Answer from the drawing. Dimensions are ordinates in mm from the lowest x, y and z of the part. A direction names the side the tool comes from. Give positions to 0.01 mm unless a question says otherwise; leave off trailing zeros. Order: outer loops, then holes, each group sorted by start corner. A loop starts at its lowest first (then second) coordinate and runs counter-clockwise, first axis right, second up.
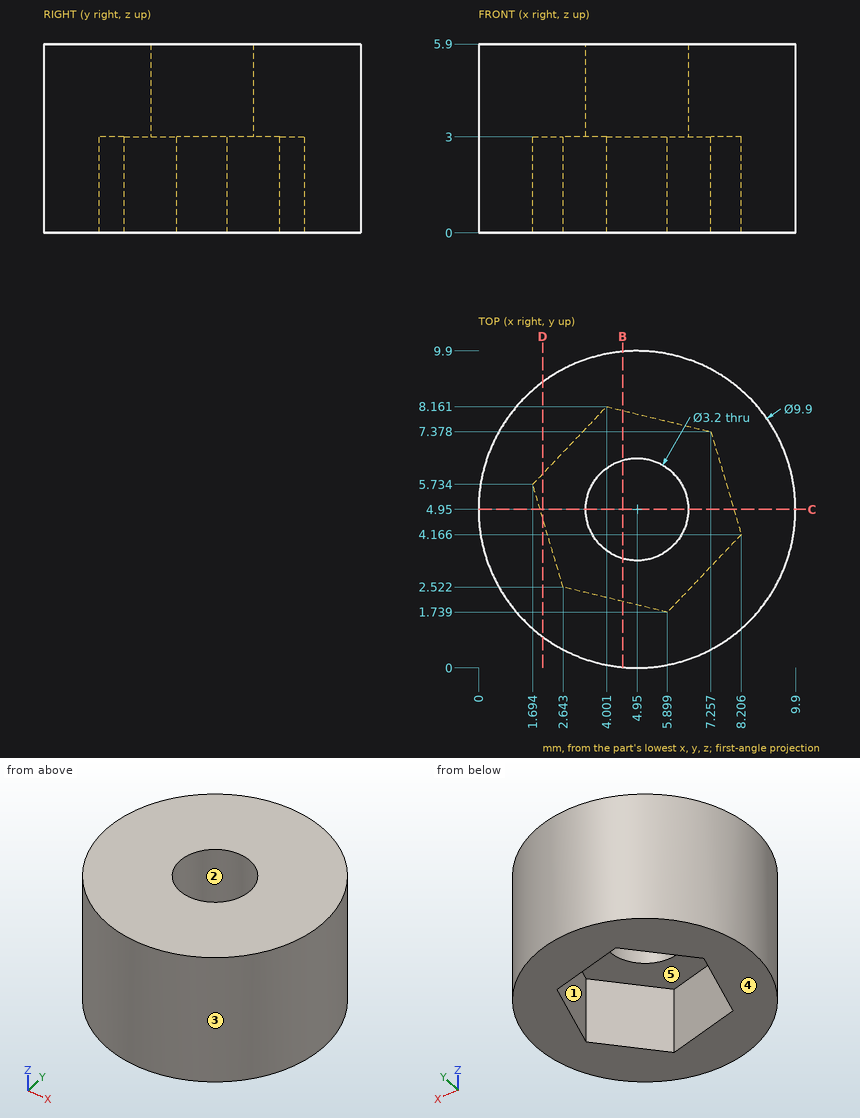
1. Given P1, Ø3, axis at x = 5, y = 4, coming from the -Z side, flat-ended and moving along its own axis, determine where the tip first touches the part or whether it passes through.
Findings below:
P1: stops at z = 3
2. Straight lines are drawn through the part: probe 1 along Y at (x, z) = (4.95, 5.25); probe 2 along Z at (x, y) = (7.25, 6). For each, find the intervals that lie inside material, in ascending order.
Findings below:
probe 1: y = 0 to 3.35, 6.55 to 9.9
probe 2: z = 3 to 5.9
3. The part is cut by section C-C (y = 4.95). Write down the section's boundary in (x, z).
Findings below:
outline: (0, 0) - (1.93, 0) - (1.93, 3) - (3.35, 3) - (3.35, 5.9) - (0, 5.9) - close; (6.55, 3) - (7.97, 3) - (7.97, 0) - (9.9, 0) - (9.9, 5.9) - (6.55, 5.9) - close
4. The part is cut by section D-D (x = 2). Write down the section's boundary in (y, z) (1 decimal).
Findings below:
outline: (1, 0) - (4.7, 0) - (4.7, 3) - (6.1, 3) - (6.1, 0) - (8.9, 0) - (8.9, 5.9) - (1, 5.9) - close
5. The part is cut by section B-B (x = 4.5). Write down the section's boundary in (y, z) (1 decimal).
Findings below:
outline: (0, 0) - (2.1, 0) - (2.1, 3) - (3.4, 3) - (3.4, 5.9) - (0, 5.9) - close; (6.5, 3) - (8, 3) - (8, 0) - (9.9, 0) - (9.9, 5.9) - (6.5, 5.9) - close
6. The mould has two halves that part along X. Classify the marked faces 3, 4 and 5: pulls with the +X half, pulls with the -X half, needs draft (parallel to the pull), parting line crosses it, or undercut.
Findings below:
face 3: parting line crosses it
face 4: needs draft
face 5: undercut
7. Which of the six approach directions +Z, -Z, +X, -X, +Y, -Y give full straight-line access (tool end or side, diameter ignored) to the marked faces 1 and 2?
Findings below:
face 1: -Z
face 2: +Z, -Z
